Read the model definition and answer for the solid it produces. Units are mm, in the model's axes. Give positions to 0.01 mm unless a question says otherwise; leave off trailing zeros. Write each loop counter-clockwise with the first axis right and the second up, starting at its lowest first coordinate (ties: lowest second). Pieces come first, ordered by that corner, then holes. Notation, with made-up numbers: (-40, 10) -> (-23, 10) arc R17 cw to (-23, 19) -> close; hole circle Ø10 at (34.25, 5.25). An arc over 180 degrees is marked (long way). Answer as CSV lines item,"result". Start each with the question number.
1. The part is cut by section B-B, the plane y = 150. Determine the outline of the cut face in (x, z).
2. Given pin 1 (1.5 mm diameter, centred on x = 3, y = 164.5, fed in from -Z); pin 2 (3 mm diameter, centred on x = 3.5, z = 448, fed in from +Y); pin 3 (1.8 mm diameter, centred on x = 4.5, z = 445.5, fed in from -Y); pin 4 (4.5 mm diameter, centred on y = 225.7, z = 413.5, fed in from +X), each flat-ended and moving along its own axis, determine where each tip first touches the part or whether it passes through.
3. Find the intervals of material crossed by line 1 (Z direction, x = 3.1, y = 241.5); line 2 (Z direction, x = 4, y = 225.7); line 3 (Y direction, x = 2.9, z = 283.51), in increasing order.
4. For a pull along Z with two mould halves and no side action, classify faces 1 (the cylindrical face through (3.042, 207.005, 354.346)), 2 (the flat face through (6, 127, 228)) as pulls with the +Z half, pulls with the -Z half, needs draft (parallel to the pull), parting line crosses it, or undercut.
5. The part is cut by section A-A, the plane x = 2.9. Give the number of separate pieces and of enclosed holes in the cut face, and give its area (3 significant figures).
from build123d import *

# Parameters (mm, degrees)
SKETCH1_W            = 450
SKETCH1_H            = 250
BOSS_EXTRUDE1_DEPTH  = 6
SKETCH2_W            = 6
SKETCH2_H            = 37.5
CUT_EXTRUDE1_DEPTH   = 515.816472153
LPATTERN1_COUNT      = 4
LPATTERN1_PITCH      = 75
LPATTERN1_COUNT_DIR2 = 2
LPATTERN1_PITCH_DIR2 = 444
SKETCH3_W            = 15
SKETCH3_H            = 6
CUT_EXTRUDE2_DEPTH   = 515.816472153
LPATTERN2_COUNT      = 2
LPATTERN2_PITCH      = 403
SKETCH4_R            = 3
CUT_EXTRUDE3_DEPTH   = 10
SKETCH5_W            = 20
SKETCH5_H            = 6
CUT_EXTRUDE4_DEPTH   = 515.816472153
SKETCH6_R            = 2.5
SKETCH6_R_2          = 2
CUT_EXTRUDE5_DEPTH   = 515.816472153


with BuildPart() as part:
    # Sketch1 → Boss-Extrude1 (new body)
    with BuildSketch(Plane(origin=(0, 0, 0), x_dir=(0, 0, -1), z_dir=(1, 0, 0))):
        with Locations((-225, 125)):
            Rectangle(SKETCH1_W, SKETCH1_H)
    extrude(amount=BOSS_EXTRUDE1_DEPTH)

    # Sketch2 → Cut-Extrude1 (cut, through all)
    with BuildSketch(Plane(origin=(6, 0, 0), x_dir=(0, 0, -1), z_dir=(1, 0, 0))):
        with Locations((-447, 231.25)):
            Rectangle(SKETCH2_W, SKETCH2_H)
    cut_extrude1 = extrude(amount=-CUT_EXTRUDE1_DEPTH, mode=Mode.SUBTRACT)

    # LPattern1: Cut-Extrude1 4 × 2
    with Locations(*[(0, -i * LPATTERN1_PITCH, -j * LPATTERN1_PITCH_DIR2) for i in range(LPATTERN1_COUNT) for j in range(LPATTERN1_COUNT_DIR2) if (i, j) != (0, 0)]):
        add(cut_extrude1, mode=Mode.SUBTRACT)

    # Sketch3 → Cut-Extrude2 (cut, through all)
    with BuildSketch(Plane(origin=(6, 0, 0), x_dir=(0, 0, -1), z_dir=(1, 0, 0))):
        with Locations((-426.5, 3)):
            Rectangle(SKETCH3_W, SKETCH3_H)
    cut_extrude2 = extrude(amount=-CUT_EXTRUDE2_DEPTH, mode=Mode.SUBTRACT)

    # LPattern2: Cut-Extrude2 ×2
    with Locations(*[(0, 0, -i * LPATTERN2_PITCH) for i in range(1, LPATTERN2_COUNT)]):
        add(cut_extrude2, mode=Mode.SUBTRACT)

    # Sketch4 → Cut-Extrude3 (cut)
    with BuildSketch(Plane(origin=(6, 0, 0), x_dir=(0, 0, -1), z_dir=(1, 0, 0))):
        with Locations((-362.5, 187)):
            Circle(SKETCH4_R)
        with Locations((-347.5, 187)):
            Circle(SKETCH4_R)
        with BuildLine():
            Line((-393.065732621, 230), (-393.065732621, 250))
            Line((-393.065732621, 250), (-316.934267379, 250))
            Line((-316.934267379, 250), (-316.934267379, 230))
            ThreePointArc((-316.934267379, 230), (-355, 207), (-393.065732621, 230))
        make_face()
    extrude(amount=-CUT_EXTRUDE3_DEPTH, mode=Mode.SUBTRACT)

    # Sketch5 → Cut-Extrude4 (cut, through all)
    with BuildSketch(Plane(origin=(6, 0, 0), x_dir=(0, 0, -1), z_dir=(1, 0, 0))):
        with Locations((-85, 3)):
            Rectangle(SKETCH5_W, SKETCH5_H)
    extrude(amount=-CUT_EXTRUDE4_DEPTH, mode=Mode.SUBTRACT)

    # Sketch6 → Cut-Extrude5 (cut, through all)
    with BuildSketch(Plane.ZY):
        with Locations((432, 225.7)):
            Circle(SKETCH6_R)
        with Locations((413.5, 225.7)):
            Circle(SKETCH6_R)
        with Locations((283.51, 241.5)):
            Circle(SKETCH6_R_2)
        with Locations((273.51, 241.5)):
            Circle(SKETCH6_R_2)
    extrude(amount=-CUT_EXTRUDE5_DEPTH, mode=Mode.SUBTRACT)


solid = part.part
Results found:
1,outline,"(0, 6) -> (6, 6) -> (6, 444) -> (0, 444) -> close"
2,pin 1,"stops at z = 6"
2,pin 2,"stops at y = 212.5"
2,pin 3,"stops at y = 25"
2,pin 4,"passes through"
3,line 1,"z = 6 to 271.51, 275.51 to 281.51, 285.51 to 316.93, 393.07 to 444"
3,line 2,"z = 6 to 319.52, 390.48 to 411, 416 to 429.5, 434.5 to 444"
3,line 3,"y = 0 to 239.5, 243.5 to 250"
4,face 1,"undercut"
4,face 2,"needs draft"
5,separate pieces,"1"
5,enclosed holes,"6"
5,area,"108,000 mm²"
